Part print with two shaded views. Sizes in mm from the minimum x, y, z corner. A direction names the side the tool comes from. Round coordinates to 2 decimals unless told otherwise and drop trailing zeros. Write each loop counter-clockwise with the first axis right and the second up, starting at its lowest first coordinate (ties: lowest second). Pieces come first, ordered by that corner, then holes. Notation, with made-up numbers: (47.25, -23) -> (69.25, -23) arc R21 ccw to (69.25, 1) -> close; hole circle Ø7 at (88, 51). An arc over 180 degrees is marked (long way). Return JSON: item names as keys, results as strings.
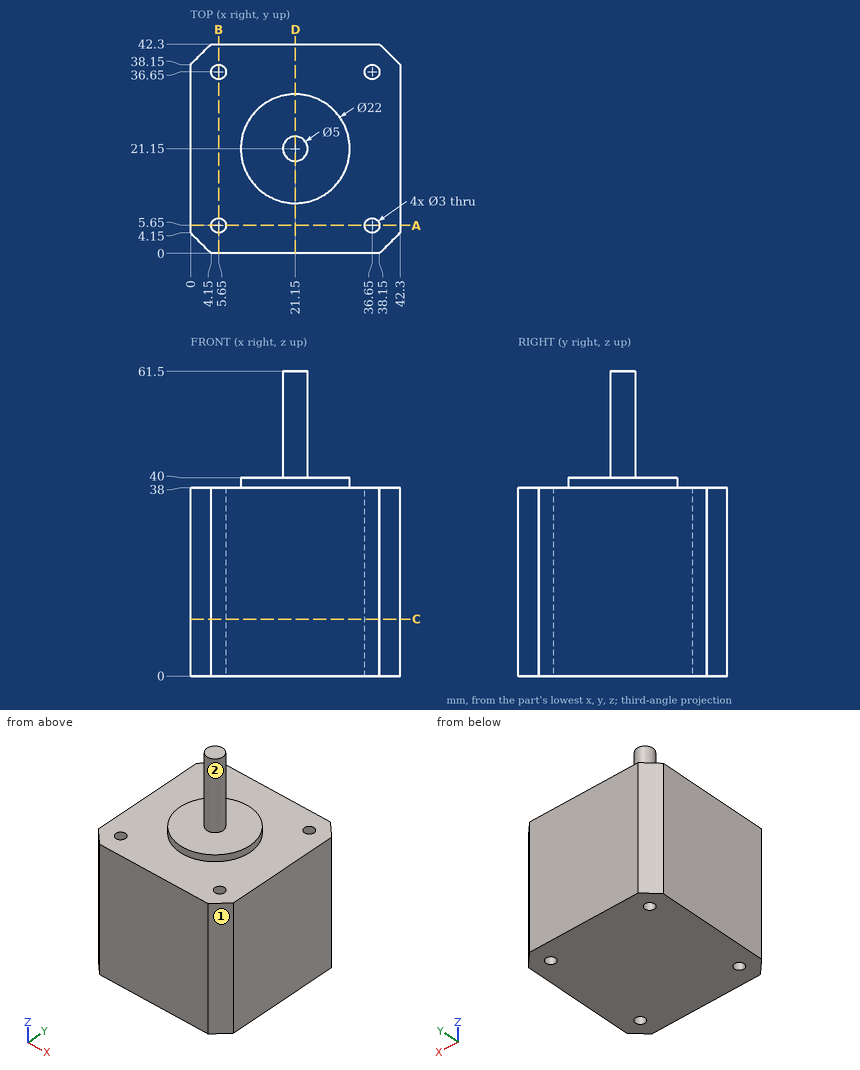
Q1. Wall check: L1, parallel to Y at x = 36.65, z = 28; L2, parallel to X at y = 5, z = 10.5. Give the ranges that are in metal, low to high.
Verdict:
{"L1": "y = 0 to 4.15, 7.15 to 35.15, 38.15 to 42.3", "L2": "x = 0 to 4.3, 7 to 35.3, 38 to 42.3"}
Q2. Saw through at C-C on z = 11.5. List the corners of the cut face in (x, y), then the cut area to 3 significant figures.
Verdict:
{"outline": "(0, 4.15) -> (4.15, 0) -> (38.15, 0) -> (42.3, 4.15) -> (42.3, 38.15) -> (38.15, 42.3) -> (4.15, 42.3) -> (0, 38.15) -> close; hole circle Ø3 at (5.65, 5.65); hole circle Ø3 at (5.65, 36.65); hole circle Ø3 at (36.65, 5.65); hole circle Ø3 at (36.65, 36.65)", "area": "1,730 mm²"}
Q3. 3-axis set-ups, long thin cutter, end or side, ignore diameter. For the marked faces 1 and 2: which of +Z, -Z, +X, -X, +Y, -Y reach the whole face in a straight line?
Verdict:
{"face 1": "+Z, -Z, +X, -Y", "face 2": "+Z"}
Q4. Pin check, flat tips, straight feed: pin 1 Ø2 at (y, z) = (34.5, 8.5) entering from -X; pin 2 Ø3.5 at (x, y) = (36.65, 5.65) entering from +Z; pin 3 Ø6.5 at (x, y) = (25, 26) entering from +Z. Stop position of each tip, or through.
Verdict:
{"pin 1": "stops at x = 0", "pin 2": "stops at z = 38", "pin 3": "stops at z = 40"}
Q5. Saw through at A-A on y = 5.65. List the corners of the cut face in (x, z), then the cut area to 3 significant figures.
Verdict:
{"outline": "(0, 0) -> (4.15, 0) -> (4.15, 38) -> (0, 38) -> close; (7.15, 0) -> (35.15, 0) -> (35.15, 38) -> (7.15, 38) -> close; (38.15, 0) -> (42.3, 0) -> (42.3, 38) -> (38.15, 38) -> close", "area": "1,380 mm²"}
Q6. Saw through at D-D on x = 21.15. List the corners of the cut face in (y, z).
Verdict:
{"outline": "(0, 0) -> (42.3, 0) -> (42.3, 38) -> (32.15, 38) -> (32.15, 40) -> (23.65, 40) -> (23.65, 61.5) -> (18.65, 61.5) -> (18.65, 40) -> (10.15, 40) -> (10.15, 38) -> (0, 38) -> close"}
